Can you work these out from the model? Positions are in its coordinate system, mm. Face numbers are marked on the shaded views. A direction names the side the tool comes from. Round coordinates to 2 decimals unless told otherwise and drop trailing zeros. Order: outer loops, then holes, each group sorted by start corner. A loop starts at its lowest first (then second) coordinate and runs counter-clockwise, first axis right, second up. Notation, with made-up numbers: M 14.25,72 L 69.25,72 A32 cw 69.25,104 Z; hole C 74.25,35 d2. An arc over 180 degrees is marked long. Answer as CSV lines item,"result". Start each with the question number.
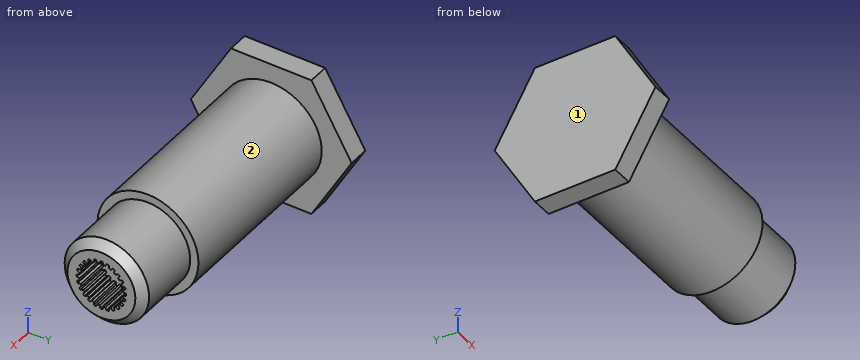
from build123d import *

# Parameters (mm, degrees)
EXTRUDE_1_DEPTH     = 2.5
CUT_EXTRUDE_1_DEPTH = 4


with BuildPart() as part:
    # Эскиз1 → Бобышка-Вытянуть1 (new body)
    with BuildSketch(Plane(origin=(0, 0, 0), x_dir=(0, 0, -1), z_dir=(1, 0, 0))):
        Polygon((0, 9.711324865), (-8.410254038, 4.855662433), (-8.410254038, -4.855662433), (0, -9.711324865), (8.410254038, -4.855662433), (8.410254038, 4.855662433), align=None)
    extrude(amount=-EXTRUDE_1_DEPTH)

    # Эскиз3 → Повернуть1 (revolve)
    with BuildSketch(Plane.XY, mode=Mode.PRIVATE) as revolve_1_sk:
        Polygon((0, 0), (0, 6.1), (22.5, 6.1), (22.5, 5.1), (30, 5.1), (31, 4.1), (31, 0), align=None)
    revolve(revolve_1_sk.sketch.rotate(Axis((-6.877569373, 0, 0), (1, 0, 0)), 90), axis=Axis((-6.877569373, 0, 0), (1, 0, 0)))

    # Эскиз4 → Вырез-Вытянуть1 (cut)
    with BuildSketch(Plane(origin=(31, 0, -31), x_dir=(0, 0, 1), z_dir=(-1, 0, 0))):
        with BuildLine():
            Line((30.778386531, 2.640717227), (30.875027145, 2.996524002))
            ThreePointArc((30.875027145, 2.996524002), (31, 2.999128925), (31.124972855, 2.996524002))
            Line((31.124972855, 2.996524002), (31.221613469, 2.640717227))
            ThreePointArc((31.221613469, 2.640717227), (31.345894409, 2.627328883), (31.469405738, 2.608094755))
            Line((31.469405738, 2.608094755), (31.654842973, 2.926765277))
            ThreePointArc((31.654842973, 2.926765277), (31.776231684, 2.896936085), (31.896271989, 2.862074568))
            Line((31.896271989, 2.862074568), (31.897530084, 2.493379183))
            ThreePointArc((31.897530084, 2.493379183), (32.014111096, 2.448280761), (32.12843572, 2.397734937))
            Line((32.12843572, 2.397734937), (32.390032334, 2.657552336))
            ThreePointArc((32.390032334, 2.657552336), (32.499564462, 2.597321838), (32.606491668, 2.532579481))
            Line((32.606491668, 2.532579481), (32.512281507, 2.176121468))
            ThreePointArc((32.512281507, 2.176121468), (32.613217787, 2.102386352), (32.710564672, 2.023973445))
            Line((32.710564672, 2.023973445), (33.030493289, 2.207231595))
            ThreePointArc((33.030493289, 2.207231595), (33.1207044, 2.1207044), (33.207231595, 2.030493289))
            Line((33.207231595, 2.030493289), (33.023973445, 1.710564672))
            ThreePointArc((33.023973445, 1.710564672), (33.102386352, 1.613217787), (33.176121468, 1.512281507))
            Line((33.176121468, 1.512281507), (33.532579481, 1.606491668))
            ThreePointArc((33.532579481, 1.606491668), (33.597321838, 1.499564462), (33.657552336, 1.390032334))
            Line((33.657552336, 1.390032334), (33.397734937, 1.12843572))
            ThreePointArc((33.397734937, 1.12843572), (33.448280761, 1.014111096), (33.493379183, 0.897530084))
            Line((33.493379183, 0.897530084), (33.862074568, 0.896271989))
            ThreePointArc((33.862074568, 0.896271989), (33.896936085, 0.776231684), (33.926765277, 0.654842973))
            Line((33.926765277, 0.654842973), (33.608094755, 0.469405738))
            ThreePointArc((33.608094755, 0.469405738), (33.627328883, 0.345894409), (33.640717227, 0.221613469))
            Line((33.640717227, 0.221613469), (33.996524002, 0.124972855))
            ThreePointArc((33.996524002, 0.124972855), (33.999128925, 0), (33.996524002, -0.124972855))
            Line((33.996524002, -0.124972855), (33.640717227, -0.221613469))
            ThreePointArc((33.640717227, -0.221613469), (33.627328883, -0.345894409), (33.608094755, -0.469405738))
            Line((33.608094755, -0.469405738), (33.926765277, -0.654842973))
            ThreePointArc((33.926765277, -0.654842973), (33.896936085, -0.776231684), (33.862074568, -0.896271989))
            Line((33.862074568, -0.896271989), (33.493379183, -0.897530084))
            ThreePointArc((33.493379183, -0.897530084), (33.448280761, -1.014111096), (33.397734937, -1.12843572))
            Line((33.397734937, -1.12843572), (33.657552336, -1.390032334))
            ThreePointArc((33.657552336, -1.390032334), (33.597321838, -1.499564462), (33.532579481, -1.606491668))
            Line((33.532579481, -1.606491668), (33.176121468, -1.512281507))
            ThreePointArc((33.176121468, -1.512281507), (33.102386352, -1.613217787), (33.023973445, -1.710564672))
            Line((33.023973445, -1.710564672), (33.207231595, -2.030493289))
            ThreePointArc((33.207231595, -2.030493289), (33.1207044, -2.1207044), (33.030493289, -2.207231595))
            Line((33.030493289, -2.207231595), (32.710564672, -2.023973445))
            ThreePointArc((32.710564672, -2.023973445), (32.613217787, -2.102386352), (32.512281507, -2.176121468))
            Line((32.512281507, -2.176121468), (32.606491668, -2.532579481))
            ThreePointArc((32.606491668, -2.532579481), (32.499564462, -2.597321838), (32.390032334, -2.657552336))
            Line((32.390032334, -2.657552336), (32.12843572, -2.397734937))
            ThreePointArc((32.12843572, -2.397734937), (32.014111096, -2.448280761), (31.897530084, -2.493379183))
            Line((31.897530084, -2.493379183), (31.896271989, -2.862074568))
            ThreePointArc((31.896271989, -2.862074568), (31.776231684, -2.896936085), (31.654842973, -2.926765277))
            Line((31.654842973, -2.926765277), (31.469405738, -2.608094755))
            ThreePointArc((31.469405738, -2.608094755), (31.345894409, -2.627328883), (31.221613469, -2.640717227))
            Line((31.221613469, -2.640717227), (31.124972855, -2.996524002))
            ThreePointArc((31.124972855, -2.996524002), (31, -2.999128925), (30.875027145, -2.996524002))
            Line((30.875027145, -2.996524002), (30.778386531, -2.640717227))
            ThreePointArc((30.778386531, -2.640717227), (30.654105591, -2.627328883), (30.530594262, -2.608094755))
            Line((30.530594262, -2.608094755), (30.345157027, -2.926765277))
            ThreePointArc((30.345157027, -2.926765277), (30.223768316, -2.896936085), (30.103728011, -2.862074568))
            Line((30.103728011, -2.862074568), (30.102469916, -2.493379183))
            ThreePointArc((30.102469916, -2.493379183), (29.985888904, -2.448280761), (29.87156428, -2.397734937))
            Line((29.87156428, -2.397734937), (29.609967666, -2.657552336))
            ThreePointArc((29.609967666, -2.657552336), (29.500435538, -2.597321838), (29.393508332, -2.532579481))
            Line((29.393508332, -2.532579481), (29.487718493, -2.176121468))
            ThreePointArc((29.487718493, -2.176121468), (29.386782213, -2.102386352), (29.289435328, -2.023973445))
            Line((29.289435328, -2.023973445), (28.969506711, -2.207231595))
            ThreePointArc((28.969506711, -2.207231595), (28.8792956, -2.1207044), (28.792768405, -2.030493289))
            Line((28.792768405, -2.030493289), (28.976026555, -1.710564672))
            ThreePointArc((28.976026555, -1.710564672), (28.897613648, -1.613217787), (28.823878532, -1.512281507))
            Line((28.823878532, -1.512281507), (28.467420519, -1.606491668))
            ThreePointArc((28.467420519, -1.606491668), (28.402678162, -1.499564462), (28.342447664, -1.390032334))
            Line((28.342447664, -1.390032334), (28.602265063, -1.12843572))
            ThreePointArc((28.602265063, -1.12843572), (28.551719239, -1.014111096), (28.506620817, -0.897530084))
            Line((28.506620817, -0.897530084), (28.137925432, -0.896271989))
            ThreePointArc((28.137925432, -0.896271989), (28.103063915, -0.776231684), (28.073234723, -0.654842973))
            Line((28.073234723, -0.654842973), (28.391905245, -0.469405738))
            ThreePointArc((28.391905245, -0.469405738), (28.372671117, -0.345894409), (28.359282773, -0.221613469))
            Line((28.359282773, -0.221613469), (28.003475998, -0.124972855))
            ThreePointArc((28.003475998, -0.124972855), (28.000871075, 0), (28.003475998, 0.124972855))
            Line((28.003475998, 0.124972855), (28.359282773, 0.221613469))
            ThreePointArc((28.359282773, 0.221613469), (28.372671117, 0.345894409), (28.391905245, 0.469405738))
            Line((28.391905245, 0.469405738), (28.073234723, 0.654842973))
            ThreePointArc((28.073234723, 0.654842973), (28.103063915, 0.776231684), (28.137925432, 0.896271989))
            Line((28.137925432, 0.896271989), (28.506620817, 0.897530084))
            ThreePointArc((28.506620817, 0.897530084), (28.551719239, 1.014111096), (28.602265063, 1.12843572))
            Line((28.602265063, 1.12843572), (28.342447664, 1.390032334))
            ThreePointArc((28.342447664, 1.390032334), (28.402678162, 1.499564462), (28.467420519, 1.606491668))
            Line((28.467420519, 1.606491668), (28.823878532, 1.512281507))
            ThreePointArc((28.823878532, 1.512281507), (28.897613648, 1.613217787), (28.976026555, 1.710564672))
            Line((28.976026555, 1.710564672), (28.792768405, 2.030493289))
            ThreePointArc((28.792768405, 2.030493289), (28.8792956, 2.1207044), (28.969506711, 2.207231595))
            Line((28.969506711, 2.207231595), (29.289435328, 2.023973445))
            ThreePointArc((29.289435328, 2.023973445), (29.386782213, 2.102386352), (29.487718493, 2.176121468))
            Line((29.487718493, 2.176121468), (29.393508332, 2.532579481))
            ThreePointArc((29.393508332, 2.532579481), (29.500435538, 2.597321838), (29.609967666, 2.657552336))
            Line((29.609967666, 2.657552336), (29.87156428, 2.397734937))
            ThreePointArc((29.87156428, 2.397734937), (29.985888904, 2.448280761), (30.102469916, 2.493379183))
            Line((30.102469916, 2.493379183), (30.103728011, 2.862074568))
            ThreePointArc((30.103728011, 2.862074568), (30.223768316, 2.896936085), (30.345157027, 2.926765277))
            Line((30.345157027, 2.926765277), (30.530594262, 2.608094755))
            ThreePointArc((30.530594262, 2.608094755), (30.654105591, 2.627328883), (30.778386531, 2.640717227))
        make_face()
    extrude(amount=CUT_EXTRUDE_1_DEPTH, mode=Mode.SUBTRACT)


solid = part.part
(1) I want a section at A-A on x = 11.5. Write out the boundary of the cut face in (y, z).
(2) I'm going to push flat-ended pins straight in: P1, Ø4, axis at x = 27.5, z = -1.5, coming from the +Y side; P2, Ø5, axis at x = 18, y = -6, coming from the -Z side; P3, Ø6, axis at x = 14, y = 1, coming from the -Z side. Where does each tip first touch, or does it pass through?
(3) For the marked faces 1 and 2, which set-ups out of +Z, -Z, +X, -X, +Y, -Y let a thin tool reach every point of the face, with its end or its side?
(4) I want a section at B-B on x = 25. Write out the boundary of the cut face in (y, z).
(5) If I drill on line 1 along X through (y, z) = (4.25, -4.5); line 2 along Y through (x, z) = (16.5, 0.25); line 3 along Y through (x, z) = (16, -5.5), over which ranges is the centre line in solid material (lowest first)?
From the geometry:
1,outline,"C 0,0 d12.2"
2,P1,"y = 5.1"
2,P2,"z = -5"
2,P3,"z = -6.1"
3,face 1,"+Z, -Z, -X, +Y, -Y"
3,face 2,"+X"
4,outline,"C 0,0 d10.2"
5,line 1,"-2.5 to 0"
5,line 2,"-6.09 to 6.09"
5,line 3,"-2.64 to 2.64"
